Could you check a few things on this drawing? It's one solid part, dimensions in mm from its lowest x, y, z. Give positions to 0.01 mm unless a question says otherwise; leave off trailing zeros. Order: outer loops, then holes, each group sorted by start corner. A loop starts at its lowest first (then second) coordinate and runs counter-clockwise, first axis right, second up. Notation, with made-up numbers: (85, -3.5) - (126, -3.5) arc R20 ccw to (126, 14.5) - close; hole circle Ø6 at (87.25, 55). An arc over 180 degrees is marked (long way). Return JSON: item names as keys, results as strings.
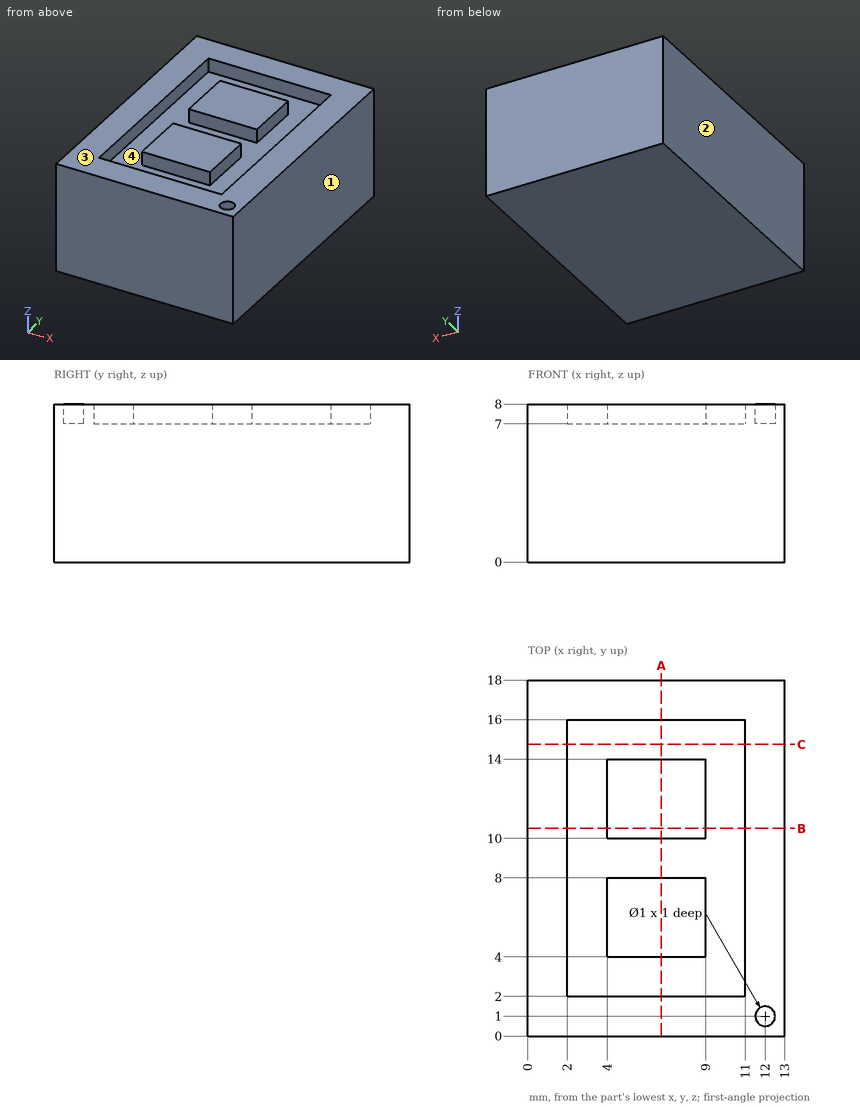
1. If I drill on L1, parallel to X at y = 13.25, z = 7.5; L2, parallel to Y at x = 12, z = 7.7; L3, parallel to Y at x = 10.25, z = 7.25, over which ranges is the centre line in solid material (lowest first)? Write a range as [from, to].
Checks:
{"L1": "[0, 2], [4, 9], [11, 13]", "L2": "[0, 0.5], [1.5, 18]", "L3": "[0, 2], [16, 18]"}
2. Thinking about a two-plate mould opening in X: for the marked faces 1, 2, 3 and 4, which applies, +X half, -X half, draft (parallel to the pull), parting line (faces both ways), or undercut?
Checks:
{"face 1": "+X half", "face 2": "-X half", "face 3": "draft", "face 4": "undercut"}
3. Suppose I cut it at A-A (x = 6.75). List the corners of the cut face in (y, z) for me.
Checks:
{"outline": "(0, 0) - (18, 0) - (18, 8) - (16, 8) - (16, 7) - (14, 7) - (14, 8) - (10, 8) - (10, 7) - (8, 7) - (8, 8) - (4, 8) - (4, 7) - (2, 7) - (2, 8) - (0, 8) - close"}
4. Suppose I cut it at C-C (y = 14.75). List the corners of the cut face in (x, z) for me, plus the area to 3 significant figures.
Checks:
{"outline": "(0, 0) - (13, 0) - (13, 8) - (11, 8) - (11, 7) - (2, 7) - (2, 8) - (0, 8) - close", "area": "95.0 mm^2"}
5. Suppose I cut it at B-B (y = 10.5). List the corners of the cut face in (x, z) for me.
Checks:
{"outline": "(0, 0) - (13, 0) - (13, 8) - (11, 8) - (11, 7) - (9, 7) - (9, 8) - (4, 8) - (4, 7) - (2, 7) - (2, 8) - (0, 8) - close"}
